Design review of the part built by this model. Coordinates are the model's own, in mm. Coordinates: 2 decimals unless noted, no trailing zeros. One line per item, written item: value.
```python
from build123d import *

# Parameters (mm, degrees)
F0_R     = 3.362501
F1_DEPTH = 215.9


with BuildPart() as f1:
    # F0 (on Top) → F1 (new body, symmetric)
    with BuildSketch(Plane.XY):
        with BuildLine():
            ThreePointArc((-7.291522, 15.377258), (-8.527575, 14.551354), (-9.985599, 14.261335))
            Line((-9.985599, 14.261335), (-12.900292, 14.261335))
            ThreePointArc((-12.900292, 14.261335), (-14.358316, 14.551354), (-15.594369, 15.377258))
            Line((-15.594369, 15.377258), (-17.43985, 17.222739))
            ThreePointArc((-17.43985, 17.222739), (-17.852803, 19.29879), (-16.092812, 20.474778))
            Line((-16.092812, 20.474778), (-14.358316, 20.474778))
            Line((-14.358316, 20.474778), (-14.325965, 20.474778))
            ThreePointArc((-14.325965, 20.474778), (-13.56835, 21.248399), (-14.325965, 22.02202))
            Line((-14.325965, 22.02202), (-14.358316, 22.02202))
            Line((-14.358316, 22.02202), (-14.996286, 22.02202))
            ThreePointArc((-14.996286, 22.02202), (-15.544549, 21.480792), (-16.092812, 22.02202))
            Line((-16.092812, 22.02202), (-19.230427, 22.02202))
            ThreePointArc((-19.230427, 22.02202), (-19.781686, 21.470761), (-20.332945, 22.02202))
            ThreePointArc((-20.332945, 22.02202), (-23.027022, 20.906097), (-24.142945, 18.21202))
            Line((-24.142945, 18.21202), (-24.142945, 17.126744))
            Line((-24.142945, 17.126744), (-24.142945, 13.971887))
            ThreePointArc((-24.142945, 13.971887), (-23.587106, 13.424695), (-24.142945, 12.877503))
            Line((-24.142945, 12.877503), (-24.142945, 12.23739))
            ThreePointArc((-24.142945, 12.23739), (-23.369324, 11.481574), (-22.595703, 12.23739))
            Line((-22.595703, 12.23739), (-22.595703, 13.971887))
            ThreePointArc((-22.595703, 13.971887), (-21.419715, 15.731877), (-19.343665, 15.318925))
            Line((-19.343665, 15.318925), (-18.091092, 14.066352))
            ThreePointArc((-18.091092, 14.066352), (-17.265188, 12.830299), (-16.975169, 11.372275))
            Line((-16.975169, 11.372275), (-16.975169, 5.601584))
            ThreePointArc((-16.975169, 5.601584), (-19.785436, 2.791317), (-22.595703, 5.601584))
            Line((-22.595703, 5.601584), (-22.595703, 6.406649))
            ThreePointArc((-22.595703, 6.406649), (-23.369324, 7.18027), (-24.142945, 6.406649))
            Line((-24.142945, 6.406649), (-24.142945, 5.771259))
            Line((-24.142945, 5.771259), (-24.142945, 1.526558))
            ThreePointArc((-24.142945, 1.526558), (-23.589161, 0.979289), (-24.142945, 0.43202))
            ThreePointArc((-24.142945, 0.43202), (-23.027022, -2.262057), (-20.332945, -3.37798))
            ThreePointArc((-20.332945, -3.37798), (-19.783762, -2.823095), (-19.234579, -3.37798))
            Line((-19.234579, -3.37798), (-15.451114, -3.37798))
            ThreePointArc((-15.451114, -3.37798), (-14.904715, -2.837846), (-14.358316, -3.37798))
            ThreePointArc((-14.358316, -3.37798), (-13.597129, -2.60328), (-14.358316, -1.82858))
            Line((-14.358316, -1.82858), (-16.090654, -1.82858))
            ThreePointArc((-16.090654, -1.82858), (-17.850645, -0.652592), (-17.437693, 1.423458))
            Line((-17.437693, 1.423458), (-15.594369, 3.266782))
            ThreePointArc((-15.594369, 3.266782), (-14.358316, 4.092686), (-12.900292, 4.382705))
            Line((-12.900292, 4.382705), (-9.985599, 4.382705))
            ThreePointArc((-9.985599, 4.382705), (-8.527575, 4.092686), (-7.291522, 3.266782))
            Line((-7.291522, 3.266782), (-5.448198, 1.423458))
            ThreePointArc((-5.448198, 1.423458), (-5.035246, -0.652592), (-6.795236, -1.82858))
            Line((-6.795236, -1.82858), (-8.527575, -1.82858))
            ThreePointArc((-8.527575, -1.82858), (-9.144781, -2.60328), (-8.527575, -3.37798))
            Line((-8.527575, -3.37798), (-7.895813, -3.37798))
            ThreePointArc((-7.895813, -3.37798), (-7.345525, -2.832718), (-6.795236, -3.37798))
            Line((-6.795236, -3.37798), (-3.641811, -3.37798))
            ThreePointArc((-3.641811, -3.37798), (-3.097378, -2.833547), (-2.552945, -3.37798))
            ThreePointArc((-2.552945, -3.37798), (0.141132, -2.262057), (1.257055, 0.43202))
            ThreePointArc((1.257055, 0.43202), (0.717674, 0.97812), (1.257055, 1.52422))
            Line((1.257055, 1.52422), (1.257055, 4.674311))
            ThreePointArc((1.257055, 4.674311), (0.713538, 5.22368), (1.257055, 5.773049))
            Line((1.257055, 5.773049), (1.257055, 6.406649))
            ThreePointArc((1.257055, 6.406649), (0.482355, 7.126711), (-0.292345, 6.406649))
            Line((-0.292345, 6.406649), (-0.292345, 4.674311))
            ThreePointArc((-0.292345, 4.674311), (-1.468333, 2.91432), (-3.544384, 3.327273))
            Line((-3.544384, 3.327273), (-5.387707, 5.170596))
            ThreePointArc((-5.387707, 5.170596), (-6.213612, 6.406649), (-6.503631, 7.864673))
            Line((-6.503631, 7.864673), (-6.503631, 10.779367))
            ThreePointArc((-6.503631, 10.779367), (-6.213612, 12.23739), (-5.387707, 13.473443))
            Line((-5.387707, 13.473443), (-3.544384, 15.316767))
            ThreePointArc((-3.544384, 15.316767), (-1.468333, 15.729719), (-0.292345, 13.969729))
            Line((-0.292345, 13.969729), (-0.292345, 12.23739))
            ThreePointArc((-0.292345, 12.23739), (0.482355, 11.501425), (1.257055, 12.23739))
            Line((1.257055, 12.23739), (1.257055, 12.877529))
            ThreePointArc((1.257055, 12.877529), (0.710955, 13.423629), (1.257055, 13.969729))
            Line((1.257055, 13.969729), (1.257055, 17.117185))
            ThreePointArc((1.257055, 17.117185), (0.705999, 17.664602), (1.257055, 18.21202))
            ThreePointArc((1.257055, 18.21202), (0.141132, 20.906097), (-2.552945, 22.02202))
            ThreePointArc((-2.552945, 22.02202), (-3.108248, 21.525639), (-3.663551, 22.02202))
            Line((-3.663551, 22.02202), (-6.793078, 22.02202))
            ThreePointArc((-6.793078, 22.02202), (-7.33931, 21.481453), (-7.885542, 22.02202))
            Line((-7.885542, 22.02202), (-8.527575, 22.02202))
            Line((-8.527575, 22.02202), (-8.599148, 22.02202))
            ThreePointArc((-8.599148, 22.02202), (-9.33781, 21.248399), (-8.599148, 20.474778))
            Line((-8.599148, 20.474778), (-8.527575, 20.474778))
            Line((-8.527575, 20.474778), (-6.793078, 20.474778))
            ThreePointArc((-6.793078, 20.474778), (-5.033088, 19.29879), (-5.44604, 17.222739))
            Line((-5.44604, 17.222739), (-7.291522, 15.377258))
        make_face()
        with Locations((-11.442945, 9.32202)):
            Circle(F0_R, mode=Mode.SUBTRACT)
        with BuildLine():
            ThreePointArc((-8.599148, 20.474778), (-8.563361, 20.473951), (-8.527575, 20.474778))
            Line((-8.527575, 20.474778), (-8.599148, 20.474778))
        make_face()
        with BuildLine():
            Line((-14.325965, 20.474778), (-14.358316, 20.474778))
            ThreePointArc((-14.358316, 20.474778), (-14.34214, 20.474609), (-14.325965, 20.474778))
        make_face()
        with BuildLine():
            ThreePointArc((-8.527575, 22.02202), (-8.563361, 22.022847), (-8.599148, 22.02202))
            Line((-8.599148, 22.02202), (-8.527575, 22.02202))
        make_face()
        with BuildLine():
            Line((-14.358316, 22.02202), (-14.325965, 22.02202))
            ThreePointArc((-14.325965, 22.02202), (-14.34214, 22.022189), (-14.358316, 22.02202))
        make_face()
    extrude(amount=F1_DEPTH, both=True)


solid = f1.part
```
(1) To check wall thickness, follow line 1 along X through (y, z) = (10, -121); line 2 along X through (y, z) = (5, -114.5); line 3 along Y through (x, z) = (-14.5, -82.5). State the ranges of each line that lie inside material, in increasing order. Write a range as [from, to].
Reply:
line 1: x = [-16.98, -14.74], [-8.15, -6.5]
line 2: x = [-24.14, -22.53], [-17.04, -5.22], [-0.29, 0.76]
line 3: y = [-3.02, -1.83], [4.03, 7.92], [10.72, 14.61], [20.47, 22.02]
(2) Mouldability with a two-part tool opening along X and no side actions: class faces 1 (the cylindrical face through (-13.921, 11.595, -3.023)), 2 (the flat face through (-14, 12, 215.9)) as released by +X, released by -X, zero draft, split by the parting line, or undercut.
Reply:
face 1: undercut
face 2: zero draft
(3) Insertion check: pin 1 (1.5 mm diameter, centred on y = -1, z = 78.5, fed in from -X); pin 2 (2.5 mm diameter, centred on x = -12, z = -83.5, fed in from +Y); pin 3 (1.5 mm diameter, centred on y = 9, z = 11.5, fed in from +X). Each pin has a flat end and moves straight along its axis. Give the tip position at first contact, or say it passes through.
Reply:
pin 1: stops at x = -24.08
pin 2: stops at y = 14.28
pin 3: stops at x = -6.5
